Geometry check sheet. Reference: the model listing, model coordinates, mm. A direction names the side the tool comes from. Coordinates: 2 decimals unless noted, no trailing zeros. Loops run counter-clockwise (first coordinate to the right, second up) from the corner with the lowest first, then second, coordinate; pieces in that order, holes last. Notation, with made-up numbers: (21.5, 24.5) -> (53.5, 24.5) arc R12 ccw to (53.5, 47.5) -> close; hole circle Ø5 at (16, 71). An arc over 180 degrees is marked (long way). Answer as a JSON object with one key per item and string values.
from build123d import *

# Parameters (mm, degrees)
SKETCH1_W               = 4.68
SKETCH1_H               = 2.52
COMPONENT_OUTLINE_DEPTH = 8.53
SKETCH2_W               = 1.4
SKETCH2_H               = 1.4
CUT_EXTRUDE1_DEPTH      = 8
LPATTERN1_COUNT         = 2
LPATTERN1_PITCH         = 2.54
SKETCH3_W               = 0.73
SKETCH3_H               = 0.5
BOSS_EXTRUDE1_DEPTH     = 3.5
LPATTERN2_COUNT         = 2
LPATTERN2_PITCH         = 2.54


with BuildPart() as part:
    # Sketch1 → Component_Outline (new body)
    with BuildSketch(Plane.XY):
        with Locations((-3.009528536, -0.057617866)):
            Rectangle(SKETCH1_W, SKETCH1_H)
    extrude(amount=COMPONENT_OUTLINE_DEPTH)

    # Sketch2 → Cut-Extrude1 (cut)
    with BuildSketch(Plane.XY.offset(8.53)):
        with Locations((-1.739528536, -0.057617866)):
            Rectangle(SKETCH2_W, SKETCH2_H)
    cut_extrude1 = extrude(amount=-CUT_EXTRUDE1_DEPTH, mode=Mode.SUBTRACT)

    # LPattern1: Cut-Extrude1 ×2
    with Locations(*[(-i * LPATTERN1_PITCH, 0, 0) for i in range(1, LPATTERN1_COUNT)]):
        add(cut_extrude1, mode=Mode.SUBTRACT)

    # Sketch3 → Boss-Extrude1 (add)
    with BuildSketch(Plane.XY.offset(0.53)):
        with Locations((-1.739528536, -0.057617866)):
            Rectangle(SKETCH3_W, SKETCH3_H)
    boss_extrude1 = extrude(amount=-BOSS_EXTRUDE1_DEPTH)

    # LPattern2: Boss-Extrude1 ×2
    with Locations(*[(-i * LPATTERN2_PITCH, 0, 0) for i in range(1, LPATTERN2_COUNT)]):
        add(boss_extrude1)


solid = part.part
1. Section check D-D, the plane y = -0.2. Record the boundary of the cut face in (x, z).
Evaluation:
{"outline": "(-5.35, 0) -> (-4.64, 0) -> (-4.64, -2.97) -> (-3.91, -2.97) -> (-3.91, 0) -> (-2.1, 0) -> (-2.1, -2.97) -> (-1.37, -2.97) -> (-1.37, 0) -> (-0.67, 0) -> (-0.67, 8.53) -> (-1.04, 8.53) -> (-1.04, 0.53) -> (-2.44, 0.53) -> (-2.44, 8.53) -> (-3.58, 8.53) -> (-3.58, 0.53) -> (-4.98, 0.53) -> (-4.98, 8.53) -> (-5.35, 8.53) -> close"}
2. Section check B-B, the plane y = 0.3. Record the boundary of the cut face in (x, z).
Evaluation:
{"outline": "(-5.35, 0) -> (-0.67, 0) -> (-0.67, 8.53) -> (-1.04, 8.53) -> (-1.04, 0.53) -> (-2.44, 0.53) -> (-2.44, 8.53) -> (-3.58, 8.53) -> (-3.58, 0.53) -> (-4.98, 0.53) -> (-4.98, 8.53) -> (-5.35, 8.53) -> close"}
3. Thickness scan on probe 1 along X at (y, z) = (0.3, 5); probe 2 along Y at (x, z) = (-1.3, 5.5); probe 3 along X at (y, z) = (-0.1, -2). Record the ranges inside material, lowest first. Write a range as from..to.
Evaluation:
{"probe 1": "x = -5.35..-4.98, -3.58..-2.44, -1.04..-0.67", "probe 2": "y = -1.32..-0.76, 0.64..1.2", "probe 3": "x = -4.64..-3.91, -2.1..-1.37"}
4. Section check C-C, the plane x = -1.2. Record the boundary of the cut face in (y, z).
Evaluation:
{"outline": "(-1.32, 0) -> (1.2, 0) -> (1.2, 8.53) -> (0.64, 8.53) -> (0.64, 0.53) -> (-0.76, 0.53) -> (-0.76, 8.53) -> (-1.32, 8.53) -> close"}
5. Tool access check on faces 5 (the face through (-5.35, 0, 4)), 6 (the face through (-2, 0, 0.53)). Record the directions out of +Z, -Z, +X, -X, +Y, -Y that give a thin tool (end or side, any length) a straight path to the whole face; none if there is none.
Evaluation:
{"face 5": "+Z, -Z, -X, +Y, -Y", "face 6": "+Z"}
6. Depth check by flat-ended pin: P1, Ø0.8, axis at x = -4.5, z = -1, coming from the +Y side; P2, Ø0.7, axis at x = -1.5, y = 0, coming from the +Z side; P3, Ø1.1, axis at x = -4, y = 0, coming from the +Z side. Enter the tip coordinate at first touch or a pass-through.
Evaluation:
{"P1": "stops at y = 0.19", "P2": "stops at z = 0.53", "P3": "stops at z = 8.53"}
7. Mould release check, pull along Y, two halves, no side actions. Record for faces 1 (the face through (-4, -0.758, 5)), 2 (the face through (-3, -1.318, 4)), 3 (the face through (-3, 0, 8.53)), 4 (the face through (-3, 1.202, 4)): released by +Y, released by -Y, zero draft, split by the parting line, or undercut.
Evaluation:
{"face 1": "undercut", "face 2": "released by -Y", "face 3": "zero draft", "face 4": "released by +Y"}
8. Section check A-A, the plane z = 1. Record the boundary of the cut face in (x, y), then the cut area to 3 significant figures.
Evaluation:
{"outline": "(-5.35, -1.32) -> (-0.67, -1.32) -> (-0.67, 1.2) -> (-5.35, 1.2) -> close; hole (-4.98, -0.76) -> (-3.58, -0.76) -> (-3.58, 0.64) -> (-4.98, 0.64) -> close; hole (-2.44, -0.76) -> (-1.04, -0.76) -> (-1.04, 0.64) -> (-2.44, 0.64) -> close", "area": "7.87 mm^2"}
